Autodesk Inventor part; units mm, degrees
ref_plane "YZ Plane" through (0, 0, 0) normal (1, 0, 0) x (0, 1, 0)
ref_plane "XZ Plane" through (0, 0, 0) normal (0, 1, 0) x (-1, 0, 0)
ref_plane "XY Plane" through (0, 0, 0) normal (0, 0, 1) x (1, 0, 0)
sketch "Szkic1" plane through (0, 0, 0) normal (0, 1, 0) x (-1, 0, 0)
  line L0 (-7.5, -7.5) -> (7.5, -7.5)
  line L1 (7.5, -7.5) -> (7.5, 7.5)
  line L2 (7.5, 7.5) -> (-7.5, 7.5)
  line L3 (-7.5, 7.5) -> (-7.5, -7.5)
  line L4 (-7.5, -7.5) -> (7.5, 7.5) construction
  line L5 (7.5, -7.5) -> (-7.5, 7.5) construction
  line L6 (6, -6) -> (-6, -6)
  line L7 (-6, -6) -> (-6, 6)
  line L8 (-6, 6) -> (6, 6)
  line L9 (6, 6) -> (6, -6)
  line L10 (6, -6) -> (-6, 6) construction
  line L11 (-6, -6) -> (6, 6) construction
  point P0 (0, 0)
  dimension "d0" = 15
  dimension "d1" = 15
  dimension "d2" = 12
  dimension "d3" = 12
extrude "Wyciągnięcie proste1" add sketch "Szkic1" along normal blind 630
sketch "Szkic2" plane through (-7.5, 0, 7.5) normal (0, 0, 1) x (1, 0, 0)
  line L0 (7.5, 0) -> (7.5, 15) construction
  dimension "d6" = 15
hole "Otwór1" at (0, 15, 7.5) direction (0, 0, -1) diameter 3.5 end through all
sketch "Szkic3" plane through (7.5, 0, 7.5) normal (1, 0, 0) x (0, 0, -1)
  line L0 (13.5, 630) -> (1.5, 630) construction
  line L1 (7.5, 630) -> (7.5, 492.75) construction
  point P0 (7.5, 0)
  dimension "d14" = 137.25
hole "Otwór2" at (7.5, 492.75, 0) direction (-1, 0, 0) diameter 3.5 end through all
sketch "Szkic4" plane through (-7.5, 0, 7.5) normal (0, 0, 1) x (1, 0, 0)
  line L0 (13.5, 630) -> (1.5, 630) construction
  line L1 (7.5, 630) -> (7.5, 590) construction
  line L2 (7.5, 630) -> (7.5, 506.5) construction
  point P0 (7.5, 0)
  dimension "d22" = 40
  dimension "d32" = 123.5
hole "Otwór3" at (0, 590, 7.5) at (0, 506.5, 7.5) direction (0, 0, -1) diameter 3.5 end through all
properties part number "bepf_glowny_wspornik" material "Aluminium 6061"
Verification items for the finished model (mm, model axes). A direction names the side the tool comes from. Round coordinates to 2 decimals unless told otherwise and drop trailing zeros. Order: outer loops, then holes, each group sorted by start corner. A loop starts at its lowest first (then second) coordinate and runs counter-clockwise, first axis right, second up.
1. Release check for a two-part mould opening along Z. For faces 1 (the flat face through (0, 311, -7.5)), 2 (the flat face through (0, 311, 7.5)), 3 (the flat face through (7.5, 311, 0)), 4 (the flat face through (6, 311, 0)) record: +Z half, -Z half, draft (parallel to the pull), parting line (faces both ways), or undercut.
Final values:
face 1: -Z half
face 2: +Z half
face 3: draft
face 4: undercut
2. Go/stop test with a flat-tipped pin: P1, Ø4, axis at x = 0, y = 590, coming from the -Z side. Record where the tip stops, or that it passes through.
Final values:
P1: stops at z = -7.5
3. Section check A-A on y = 451. Record the cut outline in (x, z), then the cut area to 3 significant figures.
Final values:
outline: (-7.5, -7.5) - (7.5, -7.5) - (7.5, 7.5) - (-7.5, 7.5) - close; hole (-6, -6) - (6, -6) - (6, 6) - (-6, 6) - close
area: 81.0 mm2
4. Access from +Z, -Z, +X, -X, +Y, -Y to the whole of each face (thin tool, end or side, straight path). Record for faces 5 (the flat face through (0, 311, 6)), 6 (the flat face through (-7.5, 311, 0)).
Final values:
face 5: +Y, -Y
face 6: +Z, -Z, -X, +Y, -Y
5. Thickness scan on L1, parallel to Y at x = 0, z = -6.6; L2, parallel to Y at x = 6.95, z = 0; L3, parallel to Z at x = -0.5, y = 524.5. Record the ranges inside material, lowest first.
Final values:
L1: y = 0 to 13.25, 16.75 to 504.75, 508.25 to 588.25, 591.75 to 630
L2: y = 0 to 491, 494.5 to 630
L3: z = -7.5 to -6, 6 to 7.5
